For this review, take the finished solid that the model builds, in its own axes (mm). A direction names the side the tool comes from. Coordinates: 2 decimals unless noted, no trailing zeros. Write each loop counter-clockwise with the first axis right and the second up, starting at its lowest first coordinate (ties: lowest second). Pieces come first, ordered by that corner, then holes.
1) For faces 5 (the face through (0.02, -7.22, 1.29)), 6 (the face through (2, 0, 0)), 7 (the face through (0, -5, 0.695)), 8 (the face through (-0.05, -3.18, -1.12)), 9 (the face through (0, -6.8, 1.3)), list the 3-axis set-ups (+Z, -Z, +X, -X, +Y, -Y) from which the entire face can be reached by the end or side of a thin tool; tool diameter is ignored.
2) We need section A-A on z = 0. Write out the cut boundary in (x, y), then the cut area to 3 significant figures.
3) We need section D-D on y = -2.25. Write out the cut boundary in (x, z).
4) Mouldability with a two-part tool opening along Y and no side actions: class faces 1 (the face through (0, 0.8, 0)), 2 (the face through (0, -6.8, -1.3)), 3 (the face through (1, -0.8, 1)), 4 (the face through (-0.02, -7.22, -1.29)) as pulls with the +Y half, pulls with the -Y half, needs draft (parallel to the pull), parting line crosses it, or undercut.
5) We need section B-B on x = 0. Write out the cut boundary in (y, z).
6) To check wall thickness, follow line 1 along Y through (x, z) = (1.25, -0.4); line 2 along Y through (x, z) = (0.15, 0.2); line 3 along Z through (x, y) = (-0.6, -6.25). State the ranges of each line that lie inside material, in increasing order.
7) Insertion check: P1, Ø2, axis at x = 0.5, y = -4, coming from the -Z side; P2, Ø1.6, axis at x = -0.5, y = -4.5, coming from the +Z side; P3, Ø1, axis at x = -1, y = -1, coming from the -Z side. Each pin has a flat end and moves straight along its axis. Give the tip position at first contact, or say it passes through.
8) We need section C-C on x = -1.4. Give the number of separate pieces and of enclosed holes in the cut face, then the cut area to 3 significant figures.
from build123d import *

# Parameters (mm, degrees)
F2_W     = 4.5
F2_H     = 1.2857143477
F3_DEPTH = 12.5
F4_R     = 0.5


with BuildPart() as f1:
    # F0 (on Right) → F1 (revolve)
    with BuildSketch(Plane.YZ):
        Polygon((-7.3752667787, 1.1195156959), (-6.8, 1.1195156959), (-6.8, 1.7445156959), align=None)
        Polygon((-7.3752667787, 0), (-0.8, 0), (-0.8, 1.1195156959), (-6.8, 1.1195156959), (-7.3752667787, 1.1195156959), align=None)
        Polygon((-0.8, 0), (0.8, 0), (0.8, 2), (-0.8, 2), (-0.8, 1.1195156959), align=None)
    revolve(axis=Axis((0, -2.8302398277, 0), (0, -1, 0)))

    # F2 (on Right) → F3 (cut, symmetric)
    with BuildSketch(Plane.YZ):
        with Locations((-5.2082390757, 0.0517627923)):
            Rectangle(F2_W, F2_H)
    extrude(amount=F3_DEPTH, both=True, mode=Mode.SUBTRACT)

    # F4
    f4_edges = [f1.edges().sort_by_distance(p)[0] for p in [
        (0, -2.958239, -0.591094),
        (0, -2.958239, 0.69462),
    ]]
    fillet(f4_edges, radius=F4_R)


solid = f1.part
Result:
1. face 5: +Z, -Y
1. face 6: +Y, -Y
1. face 7: +X, -X, -Y
1. face 8: none
1. face 9: +Z
2. outline: (-2, -0.8) - (-1.12, -0.8) - (-1.12, -2.96) - (1.12, -2.96) - (1.12, -0.8) - (2, -0.8) - (2, 0.8) - (-2, 0.8) - close
2. area: 11.2 mm2
3. outline: circle Ø2.24 at (0, 0)
4. face 1: pulls with the +Y half
4. face 2: undercut
4. face 3: undercut
4. face 4: pulls with the -Y half
5. outline: (-7.38, -1.12) - (-6.8, -1.74) - (-6.8, -1.12) - (-0.8, -1.12) - (-0.8, -2) - (0.8, -2) - (0.8, 2) - (-0.8, 2) - (-0.8, 1.12) - (-6.8, 1.12) - (-6.8, 1.74) - (-7.38, 1.12) - (-7.38, 0.69) - (-3.46, 0.69) arc R0.5 cw to (-2.96, 0.19) - (-2.96, -0.09) arc R0.5 cw to (-3.46, -0.59) - (-7.38, -0.59) - close
6. line 1: y = -0.8 to 0.8
6. line 2: y = -2.96 to 0.8
6. line 3: z = -0.95 to -0.59, 0.69 to 0.95
7. P1: stops at z = -1.12
7. P2: stops at z = 1.12
7. P3: stops at z = -1.93
8. separate pieces: 3
8. enclosed holes: 0
8. area: 4.65 mm2
